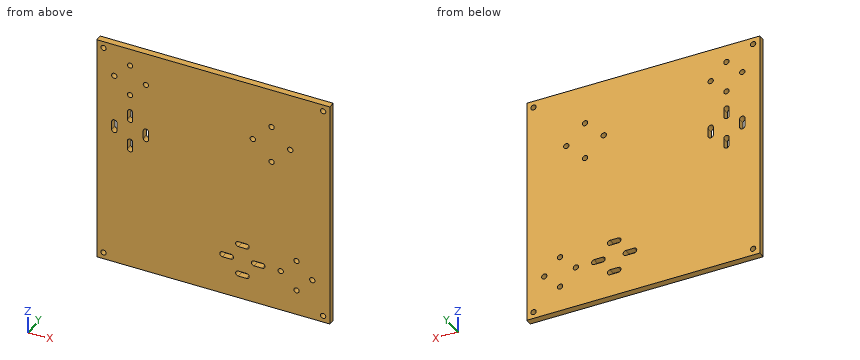
from build123d import *

# Parameters (mm, degrees)
SKETCH1_W           = 140
SKETCH1_H           = 140
BOSS_EXTRUDE1_DEPTH = 4
SKETCH2_R           = 1.6
CUT_EXTRUDE1_DEPTH  = 4
SKETCH3_R           = 1.6
CUT_EXTRUDE2_DEPTH  = 10
CUT_EXTRUDE3_DEPTH  = 10
SKETCH5_R           = 1.6
CUT_EXTRUDE5_DEPTH  = 10


with BuildPart() as part:
    # Sketch1 → Boss-Extrude1 (new body)
    with BuildSketch(Plane(origin=(0, 0, 0), x_dir=(1, 0, 0), z_dir=(0, 1, 0))):
        Rectangle(SKETCH1_W, SKETCH1_H)
    extrude(amount=BOSS_EXTRUDE1_DEPTH)

    # Sketch2 → Cut-Extrude1 (cut)
    with BuildSketch(Plane(origin=(0, 4, 0), x_dir=(1, 0, 0), z_dir=(0, 1, 0))):
        with Locations(Location((29.5, 45, 0), (0, 0, 270))):
            Circle(SKETCH2_R)
        with Locations(Location((59.5, 45, 0), (0, 0, 270))):
            Circle(SKETCH2_R)
        with Locations(Location((-50, -29.5, 0), (0, 0, 270))):
            Circle(SKETCH2_R)
        with Locations(Location((-50, -59.5, 0), (0, 0, 270))):
            Circle(SKETCH2_R)
        with Locations(Location((20, 35.5, 0), (0, 0, 270))):
            Circle(SKETCH2_R)
        with Locations(Location((10.5, 45, 0), (0, 0, 270))):
            Circle(SKETCH2_R)
        with Locations(Location((20, 54.5, 0), (0, 0, 270))):
            Circle(SKETCH2_R)
        with Locations(Location((50, 35.5, 0), (0, 0, 270))):
            Circle(SKETCH2_R)
        with Locations(Location((40.5, 45, 0), (0, 0, 270))):
            Circle(SKETCH2_R)
        with Locations(Location((50, 54.5, 0), (0, 0, 270))):
            Circle(SKETCH2_R)
        with Locations(Location((-59.5, -50, 0), (0, 0, 270))):
            Circle(SKETCH2_R)
        with Locations(Location((-50, -40.5, 0), (0, 0, 270))):
            Circle(SKETCH2_R)
        with Locations(Location((-40.5, -50, 0), (0, 0, 270))):
            Circle(SKETCH2_R)
        with Locations(Location((-59.5, -20, 0), (0, 0, 270))):
            Circle(SKETCH2_R)
        with Locations(Location((-50, -10.5, 0), (0, 0, 270))):
            Circle(SKETCH2_R)
        with Locations(Location((-40.5, -20, 0), (0, 0, 270))):
            Circle(SKETCH2_R)
    extrude(amount=-CUT_EXTRUDE1_DEPTH, mode=Mode.SUBTRACT)

    # Sketch3 → Cut-Extrude2 (cut)
    with BuildSketch(Plane(origin=(0, 4, 0), x_dir=(1, 0, 0), z_dir=(0, 1, 0))):
        with Locations(Location((35, -23.75, 0), (0, 0, 270))):
            Circle(SKETCH3_R)
        with Locations(Location((46.25, -35, 0), (0, 0, 270))):
            Circle(SKETCH3_R)
        with Locations(Location((35, -46.25, 0), (0, 0, 270))):
            Circle(SKETCH3_R)
        with Locations(Location((23.75, -35, 0), (0, 0, 270))):
            Circle(SKETCH3_R)
    extrude(amount=-CUT_EXTRUDE2_DEPTH, mode=Mode.SUBTRACT)

    # Sketch4 → Cut-Extrude3 (cut)
    with BuildSketch(Plane(origin=(0, 4, 0), x_dir=(1, 0, 0), z_dir=(0, 1, 0))):
        with BuildLine():
            Line((-51.6, -29.5), (-51.6, -24.5))
            ThreePointArc((-51.6, -24.5), (-50, -22.9), (-48.4, -24.5))
            Line((-48.4, -24.5), (-48.4, -29.5))
            ThreePointArc((-48.4, -29.5), (-50, -31.1), (-51.6, -29.5))
        make_face()
        with BuildLine():
            Line((-42.1, -20), (-42.1, -15))
            ThreePointArc((-42.1, -15), (-40.5, -13.4), (-38.9, -15))
            Line((-38.9, -15), (-38.9, -20))
            ThreePointArc((-38.9, -20), (-40.5, -21.6), (-42.1, -20))
        make_face()
        with BuildLine():
            Line((-51.6, -10.5), (-51.6, -5.5))
            ThreePointArc((-51.6, -5.5), (-50, -3.9), (-48.4, -5.5))
            Line((-48.4, -5.5), (-48.4, -10.5))
            ThreePointArc((-48.4, -10.5), (-50, -12.1), (-51.6, -10.5))
        make_face()
        with BuildLine():
            Line((-61.1, -20), (-61.1, -15))
            ThreePointArc((-61.1, -15), (-59.5, -13.4), (-57.9, -15))
            Line((-57.9, -15), (-57.9, -20))
            ThreePointArc((-57.9, -20), (-59.5, -21.6), (-61.1, -20))
        make_face()
        with BuildLine():
            Line((10.5, 43.4), (5.5, 43.4))
            ThreePointArc((5.5, 43.4), (3.9, 45), (5.5, 46.6))
            Line((5.5, 46.6), (10.5, 46.6))
            ThreePointArc((10.5, 46.6), (12.1, 45), (10.5, 43.4))
        make_face()
        with BuildLine():
            Line((20, 52.9), (15, 52.9))
            ThreePointArc((15, 52.9), (13.4, 54.5), (15, 56.1))
            Line((15, 56.1), (20, 56.1))
            ThreePointArc((20, 56.1), (21.6, 54.5), (20, 52.9))
        make_face()
        with BuildLine():
            Line((29.5, 43.4), (24.5, 43.4))
            ThreePointArc((24.5, 43.4), (22.9, 45), (24.5, 46.6))
            Line((24.5, 46.6), (29.5, 46.6))
            ThreePointArc((29.5, 46.6), (31.1, 45), (29.5, 43.4))
        make_face()
        with BuildLine():
            Line((20, 33.9), (15, 33.9))
            ThreePointArc((15, 33.9), (13.4, 35.5), (15, 37.1))
            Line((15, 37.1), (20, 37.1))
            ThreePointArc((20, 37.1), (21.6, 35.5), (20, 33.9))
        make_face()
    extrude(amount=-CUT_EXTRUDE3_DEPTH, mode=Mode.SUBTRACT)

    # Sketch5 → Cut-Extrude5 (cut)
    with BuildSketch(Plane(origin=(0, 4, 0), x_dir=(1, 0, 0), z_dir=(0, 1, 0))):
        with Locations(Location((-66, 66, 0), (0, 0, 270))):
            Circle(SKETCH5_R)
        with Locations(Location((66, 66, 0), (0, 0, 270))):
            Circle(SKETCH5_R)
        with Locations(Location((66, -66, 0), (0, 0, 270))):
            Circle(SKETCH5_R)
        with Locations(Location((-66, -66, 0), (0, 0, 270))):
            Circle(SKETCH5_R)
    extrude(amount=-CUT_EXTRUDE5_DEPTH, mode=Mode.SUBTRACT)


solid = part.part
Read the model definition and answer for the solid it produces. Units are mm, in the model's axes. Round coordinates to 2 decimals unless told otherwise and drop trailing zeros. Order: outer loops, then holes, each group sorted by start corner. A loop starts at its lowest first (then second) coordinate and runs counter-clockwise, first axis right, second up.
1) Straight lines are drawn through the part: L1, parallel to X at y = 1.55, z = 50; L2, parallel to X at y = 1.7, z = -35.5; L3, parallel to X at y = 1.8, z = 29. For each, find the intervals that lie inside material, in ascending order.
2) The part is cut by section A-A on z = 46.25. Write down the section's boundary in (x, y).
3) The part is cut by section D-D on y = 0.65. Give the number of separate pieces and of enclosed holes in the cut face, plus the area to 3 significant figures.
4) The part is cut by section C-C on z = -66. Write down the section's boundary in (x, y), plus the area to 3 significant figures.
5) The part is cut by section B-B on x = -59.5. Write down the section's boundary in (y, z).
Resolved:
1. L1: x = -70 to -61.1, -57.9 to -42.1, -38.9 to 70
1. L2: x = -70 to 13.4, 21.6 to 48.4, 51.6 to 70
1. L3: x = -70 to -51.6, -48.4 to 70
2. outline: (-70, 0) - (33.4, 0) - (33.4, 4) - (-70, 4) - close; (36.6, 0) - (70, 0) - (70, 4) - (36.6, 4) - close
3. separate pieces: 1
3. enclosed holes: 24
3. area: 19,300 mm2
4. outline: (-70, 0) - (-67.6, 0) - (-67.6, 4) - (-70, 4) - close; (-64.4, 0) - (64.4, 0) - (64.4, 4) - (-64.4, 4) - close; (67.6, 0) - (70, 0) - (70, 4) - (67.6, 4) - close
4. area: 534 mm2
5. outline: (0, -70) - (4, -70) - (4, 13.4) - (0, 13.4) - close; (0, 21.6) - (4, 21.6) - (4, 48.4) - (0, 48.4) - close; (0, 51.6) - (4, 51.6) - (4, 70) - (0, 70) - close
